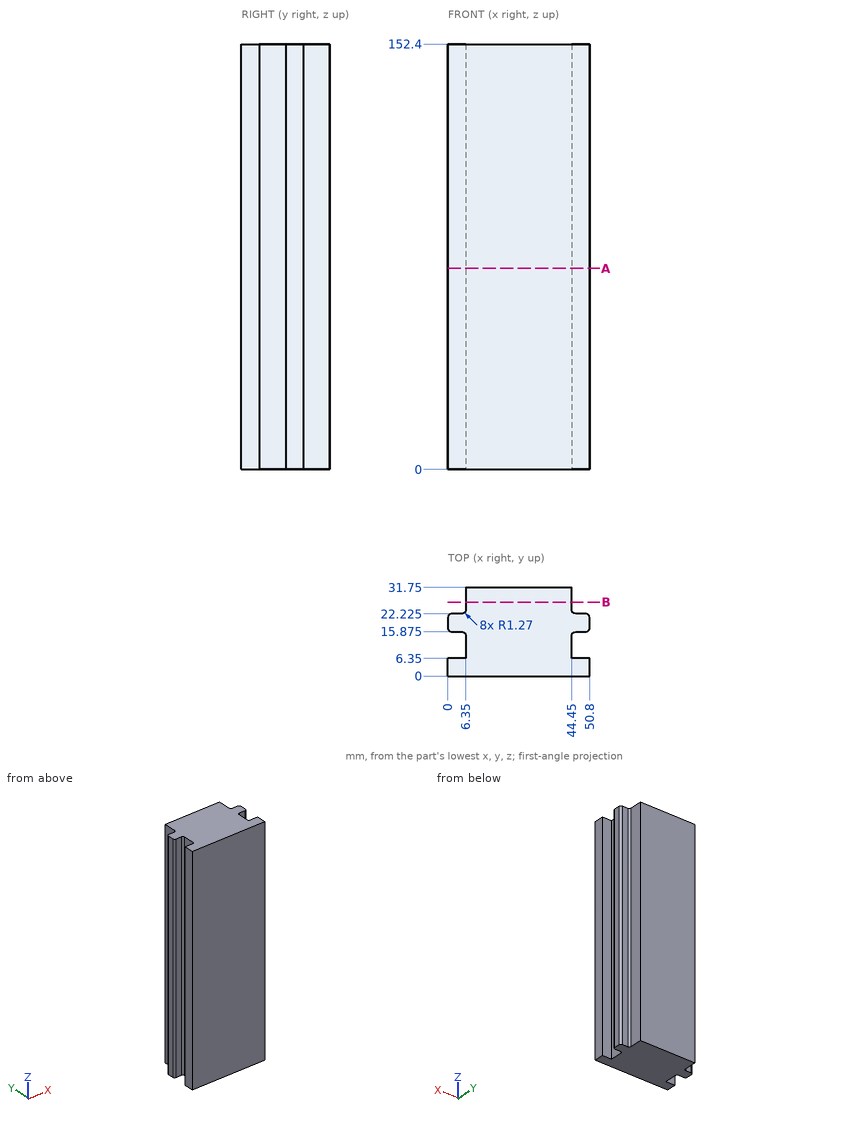
Input: dimensioned drawing with shaded views. Units: mm. Origin: part minimum x, y, z. Round coordinates to 2 decimals unless told otherwise and drop trailing zeros. Loops run counter-clockwise (first coordinate to the right, second up) from the corner with the lowest first, then second, coordinate; pieces in that order, holes last.
1) Pin query (flat end, axial travel): pin 1 (5 mm diameter, centred on x = 46, z = 49, fed in from +Y); pin 2 (1.1 mm diameter, centred on x = 3.5, z = 99.5, fed in from +Y) (3 decimals); pin 3 (9 mm diameter, centred on y = 29, z = 74, fed in from +X); pin 4 (1 mm diameter, centred on x = 45.5, z = 66, fed in from +Y). Return the tip coordinate at first contact, or that it passes through.
Ans:
pin 1: stops at y = 31.75
pin 2: stops at y = 22.225
pin 3: stops at x = 44.45
pin 4: stops at y = 22.45
2) Material intervals for line 1 (X direction, y = 26, z = 66); line 2 (Y direction, x = 45, z = 45); line 3 (X direction, y = 17, z = 106), sorted ascending.
Ans:
line 1: x = 6.35 to 44.45
line 2: y = 0 to 6.35, 15.65 to 22.45
line 3: x = 0.01 to 50.79
3) Section query A-A on z = 72. Return the cut outline in (x, y) (3 decimals).
Ans:
outline: (0, 0) - (50.8, 0) - (50.8, 6.35) - (44.45, 6.35) - (44.45, 14.605) arc R1.27 cw to (45.72, 15.875) - (49.53, 15.875) arc R1.27 ccw to (50.8, 17.145) - (50.8, 20.955) arc R1.27 ccw to (49.53, 22.225) - (45.72, 22.225) arc R1.27 cw to (44.45, 23.495) - (44.45, 31.75) - (6.35, 31.75) - (6.35, 23.495) arc R1.27 cw to (5.08, 22.225) - (1.27, 22.225) arc R1.27 ccw to (0, 20.955) - (0, 17.145) arc R1.27 ccw to (1.27, 15.875) - (5.08, 15.875) arc R1.27 cw to (6.35, 14.605) - (6.35, 6.35) - (0, 6.35) - close
4) Section query B-B on y = 26.5. Return the cut outline in (x, z), plus the area to 3 significant figures.
Ans:
outline: (6.35, 0) - (44.45, 0) - (44.45, 152.4) - (6.35, 152.4) - close
area: 5,810 mm2
